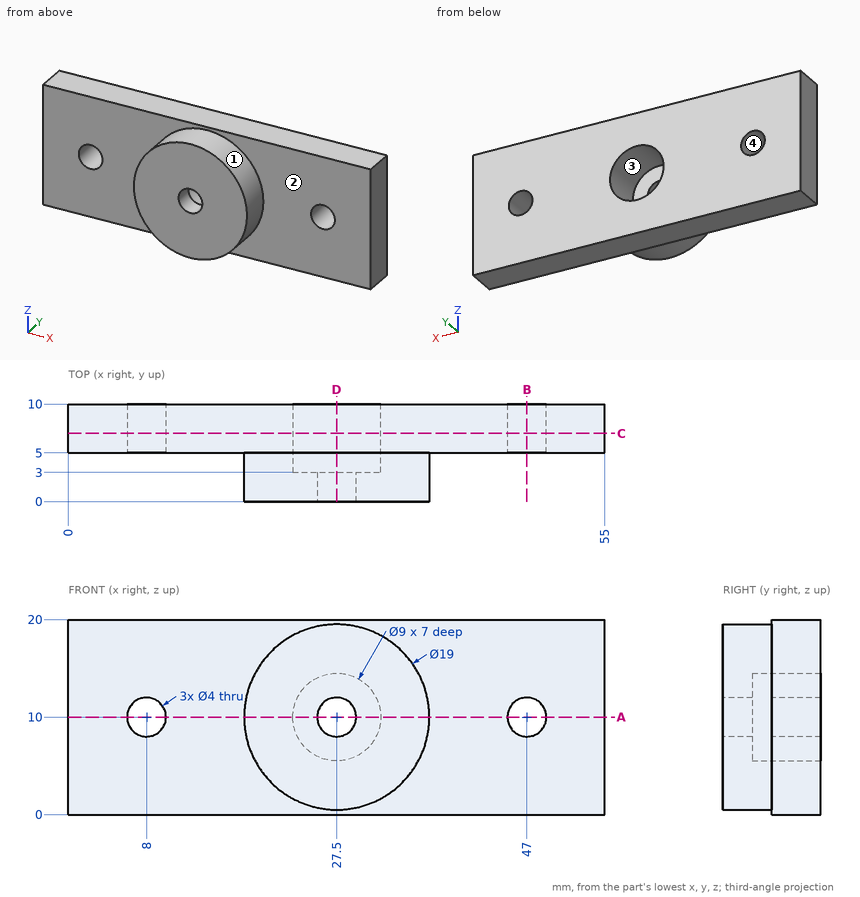
Verification items for this drawing (mm, ordinates from the low corner). Give positions to 0.01 mm unless a question says otherwise; leave off trailing zeros. Write each loop counter-clockwise with the first axis right and the second up, starting at its lowest first coordinate (ties: lowest second). Pieces come first, ordered by that corner, then holes.
1) Release check for a two-part mould opening along Z. For the marked faces 1, 2, 3 and 4 record: released by +Z, released by -Z, zero draft, split by the parting line, or undercut.
Values follow:
face 1: split by the parting line
face 2: zero draft
face 3: undercut
face 4: undercut
2) Cross-section at B-B (x = 47). Record the boundary of the cut face in (y, z).
Values follow:
outline: (5, 0) - (10, 0) - (10, 8) - (5, 8) - close; (5, 12) - (10, 12) - (10, 20) - (5, 20) - close
3) Cross-section at C-C (y = 7). Record the boundary of the cut face in (x, z), plus the area to 3 significant figures.
Values follow:
outline: (0, 0) - (55, 0) - (55, 20) - (0, 20) - close; hole circle Ø4 at (8, 10); hole circle Ø9 at (27.5, 10); hole circle Ø4 at (47, 10)
area: 1,010 mm2
4) Cross-section at D-D (x = 27.5). Record the boundary of the cut face in (y, z).
Values follow:
outline: (0, 0.5) - (5, 0.5) - (5, 0) - (10, 0) - (10, 5.5) - (3, 5.5) - (3, 8) - (0, 8) - close; (0, 12) - (3, 12) - (3, 14.5) - (10, 14.5) - (10, 20) - (5, 20) - (5, 19.5) - (0, 19.5) - close
5) Cross-section at A-A (z = 10). Record the boundary of the cut face in (x, y).
Values follow:
outline: (0, 5) - (6, 5) - (6, 10) - (0, 10) - close; (10, 5) - (18, 5) - (18, 0) - (25.5, 0) - (25.5, 3) - (23, 3) - (23, 10) - (10, 10) - close; (29.5, 0) - (37, 0) - (37, 5) - (45, 5) - (45, 10) - (32, 10) - (32, 3) - (29.5, 3) - close; (49, 5) - (55, 5) - (55, 10) - (49, 10) - close
6) Go/stop test with flat-tipped pins: pin 1 Ø5 at (x, z) = (38, 2.5) entering from -Y; pin 2 Ø7 at (x, z) = (27.5, 10) entering from +Y; pin 3 Ø4 at (y, z) = (2.5, 15) entering from +X. Record where each tip stops, or that it passes through.
Values follow:
pin 1: stops at y = 5
pin 2: stops at y = 3
pin 3: stops at x = 36.51
7) Thickness scan on line 1 (Z direction, x = 8, y = 7.45); line 2 (Z direction, x = 27.5, y = 7); line 3 (X direction, y = 8, z = 9). Record the ranges inside material, lowest first.
Values follow:
line 1: z = 0 to 8, 12 to 20
line 2: z = 0 to 5.5, 14.5 to 20
line 3: x = 0 to 6.27, 9.73 to 23.11, 31.89 to 45.27, 48.73 to 55
